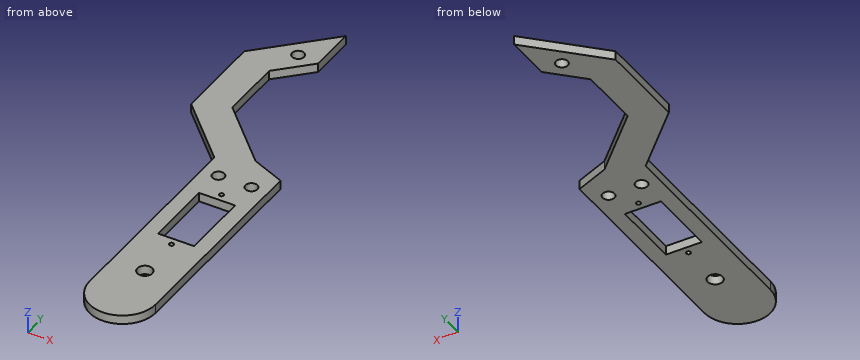
from build123d import *

# Parameters (mm, degrees)
SALIENTE_EXTRUIR1_DEPTH    = 3
CORTAR_EXTRUIR1_DEPTH      = 142.749779541
CORTAR_EXTRUIR1_DEPTH_BACK = 11
CROQUIS1_4_R               = 2
CROQUIS1_5_R               = 2
CORTAR_EXTRUIR3_DEPTH      = 142.749779541
CROQUIS1_6_W               = 12
CROQUIS1_6_H               = 23
TAMA_O_DEL_SERVO_DEPTH     = 142.749779541
CROQUIS1_7_R               = 0.75
CORTAR_EXTRUIR4_DEPTH      = 142.749779541
CROQUIS1_8_R               = 0.75
CORTAR_EXTRUIR5_DEPTH      = 142.749779541
CROQUIS1_11_R              = 2.5
CORTAR_EXTRUIR8_DEPTH      = 142.749779541


with BuildPart() as part:
    # Croquis1 → Saliente-Extruir1 (new body)
    with BuildSketch(Plane.XY):
        with BuildLine():
            Line((22, 0), (22, 70))
            Line((22, 70), (11, 74.556349186))
            Line((11, 74.556349186), (-8, 93.556349186))
            Line((-8, 93.556349186), (-8, 114.230447378))
            Line((-8, 114.230447378), (2.213203436, 124.443650814))
            Line((2.213203436, 124.443650814), (2.213203436, 140))
            Line((2.213203436, 140), (-19, 118.786796564))
            Line((-19, 118.786796564), (-19, 89))
            Line((-19, 89), (0, 70))
            Line((0, 70), (0, 0))
            ThreePointArc((0, 0), (11, -11), (22, 0))
        make_face()
    extrude(amount=SALIENTE_EXTRUIR1_DEPTH)

    # Croquis1<4> → Cortar-Extruir1 (cut, two sides: drawn at the far end of the back side and taken through both)
    with BuildSketch(Plane.XY.offset(-CORTAR_EXTRUIR1_DEPTH_BACK)):
        with Locations((5.5, 63)):
            Circle(CROQUIS1_4_R)
        with Locations((16.5, 63)):
            Circle(CROQUIS1_4_R)
    extrude(amount=CORTAR_EXTRUIR1_DEPTH + CORTAR_EXTRUIR1_DEPTH_BACK, mode=Mode.SUBTRACT)

    # Croquis1<5> → Cortar-Extruir3 (cut, through all)
    with BuildSketch(Plane.XY):
        with Locations((-4.857864376, 125.150757595)):
            Circle(CROQUIS1_5_R)
    extrude(amount=CORTAR_EXTRUIR3_DEPTH, mode=Mode.SUBTRACT)

    # Croquis1<6> → TAMAÑO DEL SERVO (cut, through all)
    with BuildSketch(Plane.XY):
        with Locations((11, 41.5)):
            Rectangle(CROQUIS1_6_W, CROQUIS1_6_H)
    extrude(amount=TAMA_O_DEL_SERVO_DEPTH, mode=Mode.SUBTRACT)

    # Croquis1<7> → Cortar-Extruir4 (cut, through all)
    with BuildSketch(Plane.XY):
        with Locations((11, 55.5)):
            Circle(CROQUIS1_7_R)
    extrude(amount=CORTAR_EXTRUIR4_DEPTH, mode=Mode.SUBTRACT)

    # Croquis1<8> → Cortar-Extruir5 (cut, through all)
    with BuildSketch(Plane.XY):
        with Locations((11, 27.5)):
            Circle(CROQUIS1_8_R)
    extrude(amount=CORTAR_EXTRUIR5_DEPTH, mode=Mode.SUBTRACT)

    # Croquis1<11> → Cortar-Extruir8 (cut, through all)
    with BuildSketch(Plane.XY):
        with Locations((11, 12.5)):
            Circle(CROQUIS1_11_R)
    extrude(amount=CORTAR_EXTRUIR8_DEPTH, mode=Mode.SUBTRACT)


solid = part.part
Here's how the part is built. I have some questions about the finished solid (model axes, mm). Give positions to 0.01 mm unless a question says otherwise; leave off trailing zeros. Order: outer loops, then holes, each group sorted by start corner. A loop starts at its lowest first (then second) coordinate and runs counter-clockwise, first axis right, second up. Notation, with made-up numbers: (-1, 18) -> (24, 18) arc R14 ccw to (24, 36) -> close; hole circle Ø4 at (-7.5, -8.5). An arc over 180 degrees is marked (long way). Use a Markdown table: item, result. Add a question column.
Item 1: Imagine slicing it at D-D on y = 95.5. Please give me the cut outline in (x, z).
Item 2: Will these pins go through, and if not, where does the flat tip stop? pin 1 (4 mm diameter, centred on x = 8, y = 71, fed in from -Z); pin 2 (0.9 mm diameter, centred on x = 11, y = 55.5, fed in from -Z); pin 3 (0.9 mm diameter, centred on y = 132, z = 1, fed in from +X); pin 4 (0.9 mm diameter, centred on y = 102, z = 2, fed in from +X).
Item 3: I need wall thicknesses on line 1 (X direction, y = 63, z = 2.2); line 2 (Y direction, x = 11, z = 1.5); line 3 (X direction, y = 12.5, z = 2.1). Which ranges of each line are inside material? Lowest first, please.
Item 4: Imagine slicing it at A-A on y = 63. Please give me the cut outline in (x, z), plus the area to 3 significant figures.
Item 5: Imagine slicing it at B-B on y = 12.5. Please give me the cut outline in (x, z).
Item 6: Imagine slicing it at C-C on z = 0.45. Please give me the cut outline in (x, y).
Data:
| question | item | result |
|---|---|---|
| 1 | outline | (-19, 0) -> (-8, 0) -> (-8, 3) -> (-19, 3) -> close |
| 2 | pin 1 | stops at z = 0 |
| 2 | pin 2 | passes through |
| 2 | pin 3 | stops at x = 2.21 |
| 2 | pin 4 | stops at x = -8 |
| 3 | line 1 | x = 0 to 3.5, 7.5 to 14.5, 18.5 to 22 |
| 3 | line 2 | y = -11 to 10, 15 to 26.75, 28.25 to 30, 53 to 54.75, 56.25 to 74.56 |
| 3 | line 3 | x = 0 to 8.5, 13.5 to 22 |
| 4 | outline | (0, 0) -> (3.5, 0) -> (3.5, 3) -> (0, 3) -> close; (7.5, 0) -> (14.5, 0) -> (14.5, 3) -> (7.5, 3) -> close; (18.5, 0) -> (22, 0) -> (22, 3) -> (18.5, 3) -> close |
| 4 | area | 42.0 mm² |
| 5 | outline | (0, 0) -> (8.5, 0) -> (8.5, 3) -> (0, 3) -> close; (13.5, 0) -> (22, 0) -> (22, 3) -> (13.5, 3) -> close |
| 6 | outline | (-19, 89) -> (0, 70) -> (0, 0) arc R11 ccw to (22, 0) -> (22, 70) -> (11, 74.56) -> (-8, 93.56) -> (-8, 114.23) -> (2.21, 124.44) -> (2.21, 140) -> (-19, 118.79) -> close; hole circle Ø4 at (-4.86, 125.15); hole circle Ø4 at (5.5, 63); hole (5, 30) -> (17, 30) -> (17, 53) -> (5, 53) -> close; hole circle Ø5 at (11, 12.5); hole circle Ø1.5 at (11, 27.5); hole circle Ø1.5 at (11, 55.5); hole circle Ø4 at (16.5, 63) |
